```python
from build123d import *

# Parameters (mm, degrees)
SKETCH1_W           = 80.01
SKETCH1_H           = 8.89
SKETCH1_R           = 2.54
BOSS_EXTRUDE1_DEPTH = 2.54
SKETCH2_W           = 8.89
SKETCH2_H           = 30.48
BOSS_EXTRUDE2_DEPTH = 2.54
SKETCH3_W           = 19.05
SKETCH3_H           = 8.89
SKETCH3_R           = 2.54
BOSS_EXTRUDE3_DEPTH = 2.54
SKETCH6_W           = 52.501867586
SKETCH6_H           = 8.89
BOSS_EXTRUDE4_DEPTH = 2.54
FILLET1_R           = 2.54


with BuildPart() as part:
    # Sketch1 → Boss-Extrude1 (new body)
    with BuildSketch(Plane(origin=(0, 0, 0), x_dir=(1, 0, 0), z_dir=(0, 1, 0))):
        with Locations((-40.005, -4.445)):
            Rectangle(SKETCH1_W, SKETCH1_H)
        with Locations((-73.66, -4.445)):
            Circle(SKETCH1_R, mode=Mode.SUBTRACT)
        with Locations((-10.16, -4.445)):
            Circle(SKETCH1_R, mode=Mode.SUBTRACT)
    extrude(amount=BOSS_EXTRUDE1_DEPTH)

    # Sketch2 → Boss-Extrude2 (add)
    with BuildSketch(Plane(origin=(0, 0, 0), x_dir=(0, 0, -1), z_dir=(1, 0, 0))):
        with Locations((-4.445, 15.24)):
            Rectangle(SKETCH2_W, SKETCH2_H)
    extrude(amount=BOSS_EXTRUDE2_DEPTH)

    # Sketch3 → Boss-Extrude3 (add)
    with BuildSketch(Plane(origin=(0, 30.48, 0), x_dir=(1, 0, 0), z_dir=(0, 1, 0))):
        with Locations((-6.985, -4.445)):
            Rectangle(SKETCH3_W, SKETCH3_H)
        with Locations((-6.985, -4.445)):
            Circle(SKETCH3_R, mode=Mode.SUBTRACT)
    extrude(amount=-BOSS_EXTRUDE3_DEPTH)

    # Sketch6 → Boss-Extrude4 (add)
    with BuildSketch(Plane(origin=(-18.408683441, 29.286541837, 0), x_dir=(0.846636549, 0.532171545, 0), z_dir=(-0.532171545, 0.846636549, 0))):
        with Locations((-24.008314522, -4.445)):
            Rectangle(SKETCH6_W, SKETCH6_H)
    extrude(amount=-BOSS_EXTRUDE4_DEPTH)

    # Fillet1
    fillet1_edges = [part.edges().sort_by_distance(p)[0] for p in [
        (2.54, 0, 4.445),
        (0, 2.54, 4.445),
        (0, 27.94, 4.445),
        (-16.51, 30.48, 4.445),
        (-15.778012038, 27.94, 4.445),
        (-56.187102947, 2.54, 4.445),
        (-60.96, 2.54, 4.445),
    ]]
    fillet(fillet1_edges, radius=FILLET1_R)


solid = part.part
```
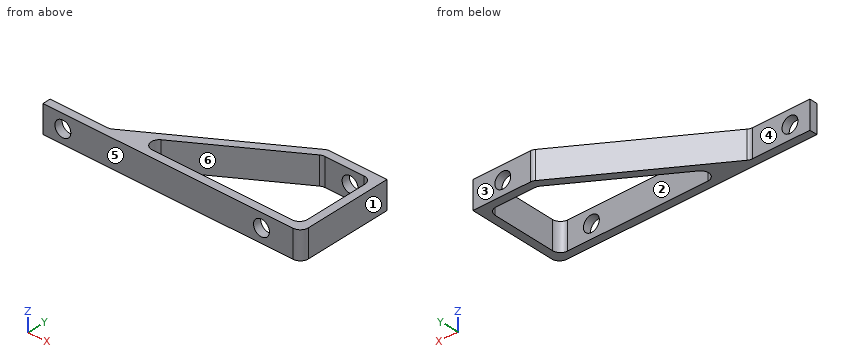
The listing builds one solid part. Answer for the finished solid, in the listing's coordinates (mm). Face numbers are marked on the shaded views. A direction names the side the tool comes from. Give positions to 0.01 mm unless a question says otherwise; leave off trailing zeros. Order: outer loops, then holes, each group sorted by start corner. A loop starts at its lowest first (then second) coordinate and runs counter-clockwise, first axis right, second up. Notation, with made-up numbers: (40.5, -7) -> (69.5, -7) arc R22 ccw to (69.5, 0) -> close; hole circle Ø9 at (54, -12). An arc over 180 degrees is marked (long way). Answer as a JSON object with one key per item and string values. Group by question number.
Item 1: Consider L1, parallel to Z at x = -10.16, y = 1.2 (3 decimals); L2, parallel to Y at x = -8, z = 1; L3, parallel to X at y = 12, z = 5.75. Determine where each line is inside the solid, lowest interval first. Write a range as from..to.
Item 2: The part is cut by section A-A on x = -73.66. Write down the section's boundary in (y, z) (3 decimals), and give its area (3 significant figures).
Item 3: The part is cut by section B-B on y = 23.5. Write down the section's boundary in (x, z), and give its area (3 significant figures).
Item 4: A tool of negligible diameter and unlimited length cuts with its end or side. For the marked faces 4, 5 and 6, from which of +Z, -Z, +X, -X, +Y, -Y can it reach the whole face along a straight path? Write none if from no direction.
Item 5: The part is cut by section D-D on x = -11. Write down the section's boundary in (y, z), and give its area (3 significant figures).
Item 6: Flat-ended cylindrical pins translate along their axes: pin 1 (3 mm diameter, centred on x = -43, z = 4, fed in from -Y); pin 2 (4 mm diameter, centred on x = -52.5, z = 5, fed in from +Y); pin 3 (1 mm diameter, centred on x = -33.5, z = 7.5, fed in from +Y); pin 4 (4.5 mm diameter, centred on y = 17, z = 5, fed in from -X) (3 decimals). Find the tip coordinate at first contact, or state that the pin passes through.
Item 7: The part is cut by section C-C on z = 5.25. Give the number of separate pieces and of enclosed holes in the cut face, and give its area (3 significant figures).
Item 8: Determine the mould class of the marked faces 1, 2 and 3 for opening direction Y: pulls with the +Y half, pulls with the -Y half, needs draft (parallel to the pull), parting line crosses it, or undercut.
Result set:
{
 "1": {"L1": "0..1.905, 6.985..8.89", "L2": "0..2.54, 27.94..30.48", "L3": "-45.91..-41.14, 0..2.54"},
 "2": {"outline": "(0, 0) -> (2.54, 0) -> (2.54, 1.905) -> (0, 1.905) -> close; (0, 6.985) -> (2.54, 6.985) -> (2.54, 8.89) -> (0, 8.89) -> close", "area": "9.68 mm²"},
 "3": {"outline": "(-27.61, 0) -> (-22.84, 0) -> (-22.84, 8.89) -> (-27.61, 8.89) -> close; (0, 0) -> (2.54, 0) -> (2.54, 8.89) -> (0, 8.89) -> close", "area": "65.0 mm²"},
 "4": {"face 4": "+Z, -Z, -X, +Y", "face 5": "+Z, -Z, +X, -X, -Y", "face 6": "+Z, -Z"},
 "5": {"outline": "(0, 0) -> (2.54, 0) -> (2.54, 2.05) -> (0, 2.05) -> close; (0, 6.84) -> (2.54, 6.84) -> (2.54, 8.89) -> (0, 8.89) -> close; (27.94, 0) -> (30.48, 0) -> (30.48, 8.89) -> (27.94, 8.89) -> close", "area": "33.0 mm²"},
 "6": {"pin 1": "y = 0", "pin 2": "y = 9.11", "pin 3": "y = 20.11", "pin 4": "x = -41.535"},
 "7": {"separate pieces": "3", "enclosed holes": "0", "area": "428 mm²"},
 "8": {"face 1": "needs draft", "face 2": "undercut", "face 3": "pulls with the +Y half"}
}
